Could you check a few things on this model? Use its own coordinates, in mm. Face numbers are marked on the shaded views. Give positions to 0.01 mm unless a question says otherwise; leave off trailing zeros. Loops run counter-clockwise (first coordinate to the right, second up) from the corner with the lowest first, then second, coordinate; pieces in that order, holes last. Notation, with made-up numbers: M 77,28.25 L 93,28.25 A17 cw 93,60.25 Z; hole C -22,25 d6. An arc over 180 degrees is marked long. Return JSON: item names as keys, results as strings. Group by question number.
1. Please list where these lines run through material, in increasing order: line 1 (Z direction, x = -3.5, y = -140); line 2 (Y direction, x = -4.3, z = -140); line 3 (Y direction, x = -8, z = -10).
2. If we section it at B-B (z = -4): Write out the boundary of the cut face in (x, y), plus the area to 4 significant figures.
3. If we section it at A-A (z = -140): State how many separate pieces and enclosed holes the cut face has, plus the area to 3 significant figures.
4. For pin 1 (6.5 mm diameter, centred on y = -140, z = -140, fed in from +X); pin 2 (2.5 mm diameter, centred on x = 15, y = -80, fed in from +Z); pin 3 (9 mm diameter, centred on x = 18.5, y = -52.5, fed in from -Z); pin 4 (6.5 mm diameter, centred on y = -140, z = -10, fed in from -X), each with a flat end and sliding along its axis, tell me the tip position at first contact or that it passes through.
5. If we mould it in two halves opening along Y, with no side actions, what happens to the marked faces 1, 2, 3 and 4? For each: +Y half, -Y half, draft (parallel to the pull), parting line (faces both ways), or undercut.
6. If we section it at C-C (x = 26.5): Write out the boundary of the cut face in (y, z), plus the area to 3 significant figures.
Autodesk Inventor part; units mm, degrees
ref_plane "YZ Plane" through (0, 0, 0) normal (1, 0, 0) x (0, 1, 0)
ref_plane "XZ Plane" through (0, 0, 0) normal (0, 1, 0) x (-1, 0, 0)
ref_plane "XY Plane" through (0, 0, 0) normal (0, 0, 1) x (1, 0, 0)
sketch "Sketch21" plane through (0, 0, 0) normal (0, 0, 1) x (1, 0, 0)
  line L0 (0, 0) -> (30, 0)
  line L1 (30, 0) -> (30, -160)
  line L2 (30, -160) -> (0, -160)
  line L3 (0, -160) -> (0, 0)
  dimension "d53" = 30
  dimension "d1" = 160
extrude "Extrusion15" add sketch "Sketch21" along normal blind 10
sketch "Sketch22" plane through (0, -160, 0) normal (-1, 0, 0) x (0, 0, 1)
  line L0 (0, 160) -> (10, 160)
  line L1 (10, 160) -> (-160, 160)
  line L2 (-160, 160) -> (-160, 0)
  line L3 (-160, 0) -> (10, 0)
  line L4 (10, 0) -> (10, 160)
  dimension "d57" = 170
  dimension "d58" = 160
extrude "Extrusion16" add sketch "Sketch22" along normal blind 10
sketch "Sketch23" plane through (30, 0, 10) normal (0, 1, 0) x (1, 0, 0)
  line L0 (-30, 170) -> (-40, 170)
  line L1 (0, 10) -> (0, 0)
  line L2 (-30, 170) -> (0, 10)
  line L3 (-30, 10) -> (0, 10)
  line L4 (0, 10) -> (-30, 10)
  line L5 (-30, 10) -> (-30, 170)
  line L6 (-40, 170) -> (-40, 0)
extrude "Extrusion17" add sketch "Sketch23" against normal blind 10
sketch "Sketch24" plane through (30, -160, 0) normal (0, -1, 0) x (1, 0, 0)
  line L0 (-30, -160) -> (-40, -160)
  line L1 (-30, 0) -> (0, 0)
  line L2 (-30, -160) -> (-30, 0)
  line L3 (0, 0) -> (0, 10)
  line L4 (-30, 0) -> (0, 0)
  line L5 (-30, -160) -> (0, 0)
  line L6 (0, 0) -> (-30, -160)
extrude "Extrusion18" add sketch "Sketch24" against normal blind 10
sketch "Sketch25" plane through (0, 0, 10) normal (0, 0, 1) x (1, 0, 0)
  circle A0 centre (15, -20) radius 1.5
  circle A1 centre (15, -80) radius 1.5
  circle A2 centre (15, -140) radius 1.5
  line L0 (30, -160) -> (-10, -160)
  line L1 (30, 0) -> (-10, 0)
  point P0 (0, 0)
  dimension "d65" = 3
  dimension "d66" = 3
  dimension "d67" = 3
  dimension "d70" = 20
  dimension "d71" = 20
  dimension "d72" = 80
extrude "Extrusion19" cut sketch "Sketch25" against normal blind 20
sketch "Sketch27" plane through (-10, -160, 0) normal (-1, 0, 0) x (0, 0, 1)
  circle A0 centre (-10, 20) radius 2
  line L0 (-160, 0) -> (10, 0)
  circle A1 centre (-10, 80) radius 2
  circle A2 centre (-10, 140) radius 2
  line L1 (10, 160) -> (-160, 160)
  line L2 (10, 0) -> (10, 160)
  circle A3 centre (-140, 80) radius 2
  line L3 (-160, 160) -> (-160, 0)
  circle A4 centre (-140, 20) radius 2
  circle A5 centre (-140, 140) radius 2
  point P0 (0, 160)
  dimension "d73" = 20
  dimension "d74" = 4
  dimension "d75" = 4
  dimension "d76" = 80
  dimension "d77" = 4
  dimension "d78" = 20
  dimension "d79" = 20
  dimension "d80" = 20
  dimension "d81" = 20
  dimension "d84" = 4
  dimension "d85" = 20
  dimension "d86" = 80
  dimension "d87" = 4
  dimension "d88" = 20
  dimension "d89" = 20
  dimension "d90" = 4
  dimension "d91" = 20
  dimension "d92" = 20
extrude "Extrusion20" cut sketch "Sketch27" against normal blind 20 contours A0 | A1 | A2 | A3 | A4 | A5
sketch "Sketch29" plane through (-10, -160, 0) normal (-1, 0, 0) x (0, 0, 1)
  circle A0 centre (-140, 80) radius 2
  circle A1 centre (-140, 80) radius 3.5
  circle A2 centre (-140, 20) radius 2
  circle A3 centre (-140, 20) radius 3.5
  circle A4 centre (-140, 140) radius 2
  circle A5 centre (-140, 140) radius 3.5
  circle A6 centre (-10, 20) radius 2
  circle A7 centre (-10, 20) radius 3.5
  circle A8 centre (-10, 80) radius 2
  circle A9 centre (-10, 80) radius 3.5
  circle A10 centre (-10, 140) radius 2
  circle A11 centre (-10, 140) radius 3.5
  point P0 (0, 160)
  dimension "d93" = 7
  dimension "d94" = 7
  dimension "d95" = 7
  dimension "d96" = 7
  dimension "d97" = 7
  dimension "d98" = 7
extrude "Extrusion21" cut sketch "Sketch29" against normal blind 4 contours A0 | A1 | A2 | A3 | A4 | A5 | A6 | A7 | A8 | A9 | A10 | A11
equation "\"d58\" = d1"
equation "\"d65\" = d67"
equation "\"d66\" = d67"
equation "\"d71\" = d70"
equation "\"d73\" = d70"
equation "\"d74\" = d75"
equation "\"d76\" = d72"
equation "\"d77\" = d75"
equation "\"d78\" = d70"
equation "\"d80\" = d79"
equation "\"d81\" = d79"
equation "\"d84\" = d75"
equation "\"d85\" = d79"
equation "\"d86\" = d72"
equation "\"d87\" = d75"
equation "\"d88\" = d79"
equation "\"d89\" = d70"
equation "\"d90\" = d75"
equation "\"d91\" = d79"
equation "\"d92\" = d70"
equation "\"d94\" = d93"
equation "\"d95\" = d93"
equation "\"d96\" = d93"
equation "\"d97\" = d93"
equation "\"d98\" = d93"
properties part number "bracket_v01"
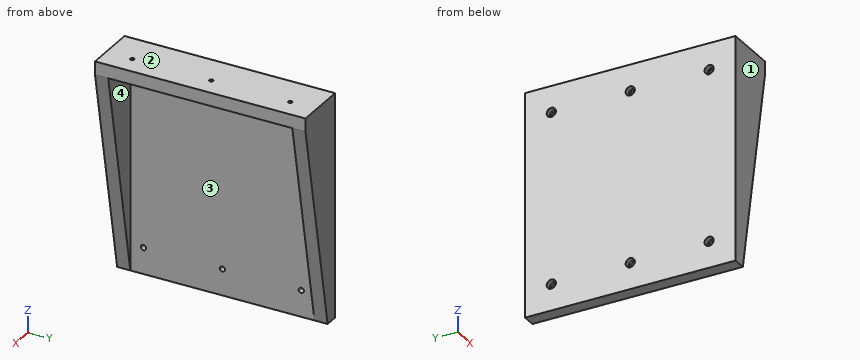
Answer:
{
 "1": {"line 1": "z = -160 to -142, -138 to -12, -8 to 10", "line 2": "y = -160 to -142, -138 to -82, -78 to -22, -18 to 0", "line 3": "y = -160 to -143.5, -136.5 to -83.5, -76.5 to -23.5, -16.5 to 0"},
 "2": {"outline": "M -10,-160 L 29.25,-160 L 29.25,-150 L 0,-150 L 0,-10 L 29.25,-10 L 29.25,0 L -10,0 Z", "area": "2,185 mm²"},
 "3": {"separate pieces": "4", "enclosed holes": "0", "area": "1,520 mm²"},
 "4": {"pin 1": "stops at x = 0", "pin 2": "passes through", "pin 3": "stops at z = 0", "pin 4": "stops at x = -6"},
 "5": {"face 1": "-Y half", "face 2": "draft", "face 3": "undercut", "face 4": "undercut"},
 "6": {"outline": "M -160,-18.67 L -150,-18.67 L -150,0 L -10,0 L -10,-18.67 L 0,-18.67 L 0,10 L -160,10 Z", "area": "1,970 mm²"}
}
